Here's how the part is built. I have some questions about the finished solid (model axes, mm). Face numbers are marked on the shaded views. A direction names the side the tool comes from. Round coordinates to 2 decimals unless told otherwise and drop trailing zeros. Loops run counter-clockwise (first coordinate to the right, second up) from the corner with the lowest first, then second, coordinate; pieces in that order, holes last. Notation, with made-up numbers: M 24,76 L 65,76 A18 cw 65,97 Z; hole C -6.75,39.5 d3. An arc over 180 degrees is marked long. One line per question, with ' | ' between items. Start each with the question number.
```python
from build123d import *

# Parameters (mm, degrees)
F0_W     = 30
F0_H     = 316
F1_DEPTH = 5
F2_DEPTH = 17.5
F3_SIZE2 = 14.99999
F3_SIZE  = 22.49999
F4_SIZE2 = 22.49999
F4_SIZE  = 29.99999
F5_T     = 2.5
F6_DEPTH = 2.4
F7_DEPTH = 25


# Not quite as in the source:
# - a fillet or chamfer is up to 0.001 mm smaller than in the source, because OpenCascade refuses the exact size
# - a shell that OpenCascade refuses in one call is made with other operations: the cavity is built on its own and cut out


with BuildPart() as f1:
    # F0 (on Top) → F1 (new body)
    with BuildSketch(Plane.XY):
        Rectangle(F0_W, F0_H)
    extrude(amount=F1_DEPTH)

    # F2 (add): a face of the model
    f2_faces = [f1.faces().sort_by_distance(p)[0] for p in [
        (0, 0, 0),
    ]]
    extrude(f2_faces, amount=F2_DEPTH)

    # F3 (size 22.5 and 15 in the source; OpenCascade refuses exactly that, so slightly less here)
    f3_edges = [f1.edges().sort_by_distance(p)[0] for p in [
        (0, 158, 5),
    ]]
    f3_side = f1.faces().sort_by_distance((0, 158, -6.25))[0]
    chamfer(f3_edges, length=F3_SIZE, length2=F3_SIZE2, reference=f3_side)

    # F4 (size 30 and 22.5 in the source; OpenCascade refuses exactly that, so slightly less here)
    f4_edges = [f1.edges().sort_by_distance(p)[0] for p in [
        (0, -158, 5),
    ]]
    f4_side = f1.faces().sort_by_distance((0, -7.499995, 5))[0]
    chamfer(f4_edges, length=F4_SIZE, length2=F4_SIZE2, reference=f4_side)

    # F5: shell of thickness 2.5, made by hand


with BuildPart() as f5_core1:
    # F5_t2: copy of F1
    add(f1.part)

    # the walls: a layer under each face that stays
    f5_faces = [f5_core1.faces().sort_by_distance(p)[0] for p in [
        (15, 0, -6.25),
        (0, 7.5, 5),
        (0, -143.000005, -6.249995),
        (0, 150.500005, -6.249995),
        (0, -158, -17.499995),
        (0, 158, -17.499995),
        (-15, 0, -6.25),
    ]]
    thicken(f5_faces, amount=-F5_T, mode=Mode.SUBTRACT)


with BuildPart() as f1_1:
    add(f1.part)

    # what is left inside the walls is the cavity
    f5_cavity = [f5_core1.part.solids().sort_by_distance(p)[0] for p in [
        (0, -50.890437, -17.475),
    ]]
    add(f5_cavity, mode=Mode.SUBTRACT)

    # F6 (cut): a face of the model
    f6_faces = [f1_1.faces().sort_by_distance(p)[0] for p in [
        (-12.5, 3.8374129004, -7.7308172989),
    ]]
    extrude(f6_faces, amount=-F6_DEPTH, mode=Mode.SUBTRACT)

    # F7 (cut): a face of the model
    f7_faces = [f1_1.faces().sort_by_distance(p)[0] for p in [
        (12.5, 3.8374129004, -7.7308172989),
    ]]
    extrude(f7_faces, amount=-F7_DEPTH, mode=Mode.SUBTRACT)


solid = f1_1.part
```
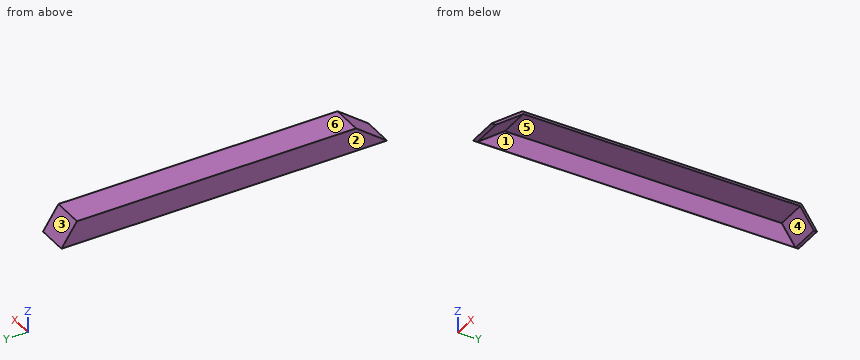
1) I'm going to push flat-ended pins straight in: pin 1 Ø6 at (y, z) = (-21, -10) entering from +X; pin 2 Ø10 at (x, z) = (-7, -7.5) entering from +Y; pin 3 Ø6 at (x, y) = (5, 60) entering from -Z. Where does each tip first touch, or does it pass through?
2) Imagine slicing it at B-B (y = -29). Write out the boundary of the cut face in (x, z), then the cut area to 3 significant figures.
3) For the marked faces 1 and 2, which set-ups out of +Z, -Z, +X, -X, +Y, -Y let a thin tool reach every point of the face, with its end or its side?
4) Imagine slicing it at C-C (z = -4). Write out the boundary of the cut face in (x, y), then the cut area to 3 significant figures.
5) Please list where these lines run through material, in increasing order: L1, parallel to Z at x = -3, y = 126; L2, parallel to Y at x = -13.75, z = -2; L3, parallel to Y at x = 3, z = -5.25. Write a range as from..to.
6) We'd pull the mould along Y, two halves only. Please class the marked faces 3, 4, 5 and 6: pulls with the +Y half, pulls with the -Y half, needs draft (parallel to the pull), parting line crosses it, or undercut.
Results are:
1) pin 1: x = -14.9 | pin 2: y = 154.67 | pin 3: z = 2.5
2) outline: M -15,-17.5 L -14.9,-17.5 L -14.9,2.5 L 15,2.5 L 15,5 L -15,5 Z | area: 77.0 mm²
3) face 1: -Z, +X | face 2: +Z, -Z, -X, +Y, -Y
4) outline: M -15,-140 L 15,-140 L 15,-135.83 L -14.9,-135.83 L -14.9,146 L 15,146 L 15,149 L -15,149 Z | area: 243 mm²
5) L1: 2.5..5 | L2: -137.33..-133.17, 144.66..147.67 | L3: -141.67..-137.5, 146.83..149.83
6) face 3: pulls with the +Y half | face 4: undercut | face 5: undercut | face 6: needs draft
